Input: dimensioned drawing with shaded views. Units: mm. Origin: part minimum x, y, z. Give positions to 0.01 mm unless a question says otherwise; leave off trailing zeros. Loops run counter-clockwise (first coordinate to the right, second up) from the corner with the lowest first, then second, coordinate; pieces in that order, holes last.
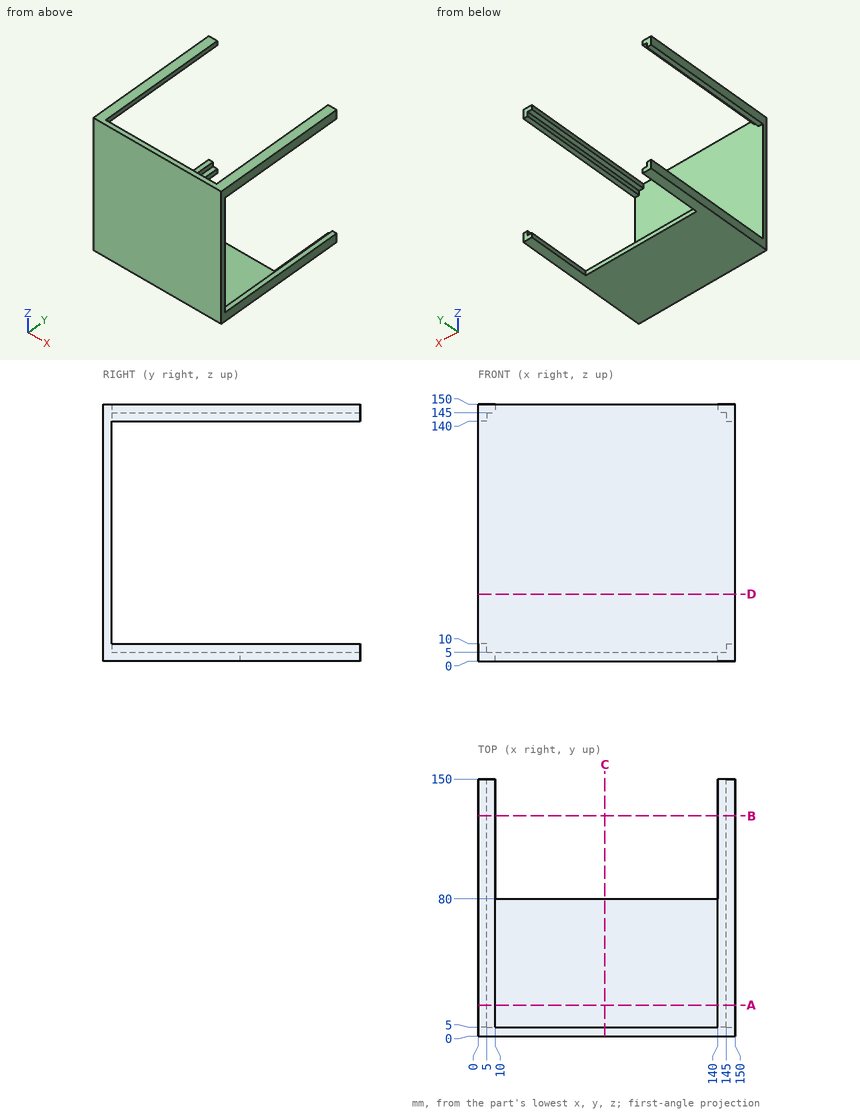
Item 1: Pin query (flat end, axial travel): pin 1 (2 mm diameter, centred on x = 34.5, z = 35.5, fed in from +Y); pin 2 (12 mm diameter, centred on x = 102.5, y = 88.5, fed in from -Z); pin 3 (3 mm diameter, centred on x = 23.5, y = 37, fed in from +Z). Return the tip coordinate at first contact, or that it passes through.
Values follow:
pin 1: stops at y = 5
pin 2: passes through
pin 3: stops at z = 5
Item 2: Section query C-C on x = 74. Return loops of the section in (y, z).
Values follow:
outline: (0, 0) - (80, 0) - (80, 5) - (5, 5) - (5, 150) - (0, 150) - close
Item 3: Section query D-D on z = 39. Return loops of the section in (x, y).
Values follow:
outline: (0, 0) - (150, 0) - (150, 5) - (0, 5) - close
Item 4: Section query B-B on y = 128.5. Return loops of the section in (x, z).
Values follow:
outline: (0, 0) - (10, 0) - (10, 5) - (5, 5) - (5, 10) - (0, 10) - close; (0, 140) - (5, 140) - (5, 145) - (10, 145) - (10, 150) - (0, 150) - close; (140, 0) - (150, 0) - (150, 10) - (145, 10) - (145, 5) - (140, 5) - close; (140, 145) - (145, 145) - (145, 140) - (150, 140) - (150, 150) - (140, 150) - close
Item 5: Section query A-A on y = 18. Return loops of the section in (x, z), plus the area to 3 significant figures.
Values follow:
outline: (0, 0) - (150, 0) - (150, 10) - (145, 10) - (145, 5) - (5, 5) - (5, 10) - (0, 10) - close; (0, 140) - (5, 140) - (5, 145) - (10, 145) - (10, 150) - (0, 150) - close; (140, 145) - (145, 145) - (145, 140) - (150, 140) - (150, 150) - (140, 150) - close
area: 950 mm2
Item 6: Ray query, probe 1 along Z at (x, y) = (8.5, 87); probe 2 along Z at (x, y) = (106.5, 36). Return the intervals inside material, ascending.
Values follow:
probe 1: z = 0 to 5, 145 to 150
probe 2: z = 0 to 5
